Can you work these out from the model? Positions are in its coordinate system, mm. Face numbers are marked on the shaded views. A direction names the side the tool comes from. Give positions to 0.01 mm unless a question says otherwise; leave off trailing zeros. Order: outer loops, then holes, each group sorted by start corner. A loop starts at its lowest first (then second) coordinate and runs counter-clockwise, first axis right, second up. Notation, with made-up numbers: (79.25, 70) -> (132.25, 70) arc R20 cw to (132.25, 90) -> close; hole circle Ø5 at (-38, 8). An arc over 180 degrees is marked (long way). Answer as a JSON object with one key per item and string values.
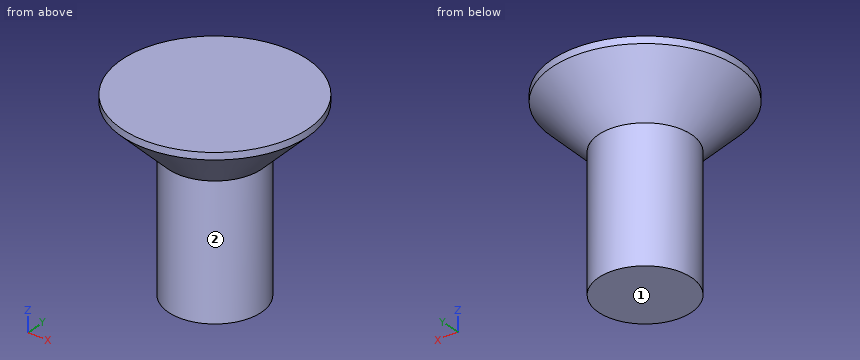
Autodesk Inventor part; units mm, degrees
ref_plane "YZ Plane" through (0, 0, 0) normal (1, 0, 0) x (0, 1, 0)
ref_plane "XZ Plane" through (0, 0, 0) normal (0, 1, 0) x (-1, 0, 0)
ref_plane "XY Plane" through (0, 0, 0) normal (0, 0, 1) x (1, 0, 0)
sketch "スケッチ1" plane through (0, 0, 0) normal (0, 0, 1) x (1, 0, 0)
  circle A0 centre (0, 0) radius 2
  dimension "d0" = 4
extrude "押し出し1" add sketch "スケッチ1" along normal blind 6
sketch "スケッチ2" plane through (0, 0, 6) normal (0, 0, 1) x (1, 0, 0)
  circle A0 centre (0, 0) radius 2
  circle A1 centre (0, 0) radius 4
  dimension "d3" = 8
extrude "押し出し2" add sketch "スケッチ2" along normal blind 2.3 contours A0 | A1
thread "ねじ1"
sketch "スケッチ3" plane through (0, 0, 0) normal (0, 0, -1) x (-1, 0, 0)
  circle A0 centre (0, 0) radius 2
extrude "押し出し3" cut sketch "スケッチ3" against normal blind 0.3
chamfer "面取り1" distance 2 angle 45 1 edges at (-4, 0, 6)
properties part number "SB　M4 8mm 皿ネジ" material "Stainless Steel, 440C"
1. If we section it at D-D on z = 6.5: Please give me the cut outline in (x, y), then the cut area to 3 significant figures.
Worked answers:
{"outline": "circle Ø5 at (0, 0)", "area": "19.6 mm²"}
2. For the marked faces 1 and 2, which set-ups out of +Z, -Z, +X, -X, +Y, -Y let a thin tool reach every point of the face, with its end or its side?
Worked answers:
{"face 1": "-Z, +X, -X, +Y, -Y", "face 2": "-Z"}
3. If we section it at C-C on z = 3.25: Please give me the cut outline in (x, y).
Worked answers:
{"outline": "circle Ø4 at (0, 0)"}
4. Please list where these lines run through material, in increasing order: L1, parallel to Y at x = 1, z = 8.25; L2, parallel to Y at x = 2, z = 6.5; L3, parallel to Z at x = -1.75, y = 1.5.
Worked answers:
{"L1": "-3.87 to 3.87", "L2": "-1.5 to 1.5", "L3": "6.3 to 8.3"}
5. Will these pins go through, and if not, where does the flat tip stop? pin 1 Ø1 at (y, z) = (3, 6) entering from +X; pin 2 Ø4 at (x, z) = (1, 4) entering from -Y; pin 3 Ø1.5 at (x, z) = (0, 7) entering from +Y; pin 4 Ø1 at (x, z) = (0.5, 6.5) entering from +Y.
Worked answers:
{"pin 1": "through", "pin 2": "y = -2", "pin 3": "y = 3.75", "pin 4": "y = 2.96"}
